Geometry: final body of the model. Coordinates: model frame, mm. A direction names the side the tool comes from. Round coordinates to 2 decimals unless told otherwise and drop trailing zeros. Write each loop counter-clockwise with the first axis right and the second up, starting at its lowest first coordinate (ties: lowest second). Pieces come first, ordered by that corner, then holes. Notation, with made-up numbers: M 24.25,79.25 L 80.25,79.25 A25 ccw 80.25,96.25 Z; hole C 71,2.5 d6. An arc over 180 degrees is marked long. Answer as CSV lines item,"result". Start each with the question number.
Q1. First-contact query: pin 1 (3 mm diameter, centred on x = 0.5, z = 3, fed in from -Y) (3 decimals); pin 2 (1.5 mm diameter, centred on x = 2.5, z = 2.5, fed in from +Y). Flat tips, straight axial feed; report the tip coordinate or a pass-through.
Q2. Reachability of faces 1 (the flat face through (1, -1, 5)), 2 (the cylindrical face through (-1.57, -1.2, 3.32)) from +Z, -Z, +X, -X, +Y, -Y: full face, straight path, thin tool, end or side. Return the list, or none.
Q3. Section query D-D on z = 0.75. Output: boundary loops of the cut face in (x, y) (3 decimals), and give its area (3 significant figures).
Q4. Section query C-C on z = 2.35. Output: boundary loops of the cut face in (x, y) (3 decimals).
Q5. Ray query, probe 1 along Y at (x, z) = (0, 2.6) (3 decimals); probe 2 along Y at (x, z) = (-0.25, 1.45); probe 3 along Z at (x, y) = (-1.5, -1.75). Return the intervals inside material, ascending.
Q6. Section query A-A on x = 0. Output: boundary loops of the cut face in (y, z) (3 decimals), and give its area (3 significant figures).
```python
from build123d import *

# Parameters (mm, degrees)
ESBO_O1_R                = 1.975
ESBO_O1_R_2              = 1.175
RESSALTO_EXTRUS_O1_DEPTH = 5
ESBO_O2_R                = 3.765
ESBO_O2_R_2              = 1.175
RESSALTO_EXTRUS_O2_DEPTH = 1.68
CHANFRO1_SIZE            = 1.4


with BuildPart() as part:
    # Esboço1 → Ressalto-extrusão1 (new body)
    with BuildSketch(Plane.XY):
        Circle(ESBO_O1_R)
        Circle(ESBO_O1_R_2, mode=Mode.SUBTRACT)
    extrude(amount=RESSALTO_EXTRUS_O1_DEPTH)

    # Esboço2 → Ressalto-extrusão2 (add)
    with BuildSketch(Plane(origin=(0, 0, 0), x_dir=(-1, 0, 0), z_dir=(0, 0, -1))):
        Circle(ESBO_O2_R)
        with Locations(Location((0, 0, 0), (0, 0, 180))):
            Circle(ESBO_O2_R_2, mode=Mode.SUBTRACT)
    extrude(amount=-RESSALTO_EXTRUS_O2_DEPTH)

    # Chanfro1
    chanfro1_edges = [part.edges().sort_by_distance(p)[0] for p in [
        (3.765, 0, 0),
    ]]
    chamfer(chanfro1_edges, length=CHANFRO1_SIZE)


solid = part.part
```
Entries:
1,pin 1,"stops at y = -3.765"
1,pin 2,"stops at y = 0.92"
2,face 1,"+Z, +X, -X, +Y, -Y"
2,face 2,"+Z"
3,outline,"C 0,0 d6.23; hole C 0,0 d2.35"
3,area,"26.1 mm^2"
4,outline,"C 0,0 d3.95; hole C 0,0 d2.35"
5,probe 1,"y = -1.975 to -1.175, 1.175 to 1.975"
5,probe 2,"y = -3.76 to -1.15, 1.15 to 3.76"
5,probe 3,"z = 0 to 1.68"
6,outline,"M -3.765,1.4 L -2.365,0 L -1.175,0 L -1.175,5 L -1.975,5 L -1.975,1.68 L -3.765,1.68 Z; M 1.175,0 L 2.365,0 L 3.765,1.4 L 3.765,1.68 L 1.975,1.68 L 1.975,5 L 1.175,5 Z"
6,area,"12.1 mm^2"
